For this review, take the finished solid that the model builds, in its own axes (mm). Face numbers are marked on the shaded views. A direction names the side the tool comes from. Give positions to 0.01 mm unless a question says otherwise; leave off trailing zeros. Order: outer loops, then holes, each group sorted by start corner. A loop starts at its lowest first (then second) coordinate and runs counter-clockwise, first axis right, second up. Notation, with made-up numbers: (-6, 8.25) -> (21, 8.25) arc R10 cw to (21, 18.25) -> close; hole circle Ø9 at (29, 70.5). An arc over 180 degrees is marked (long way). Return JSON: item names as keys, results as strings. Group by question number.
1) Insertion check: P1, Ø3.5, axis at x = -1.5, z = -1.5, coming from the +Y side; P2, Ø1.5, axis at y = 10.5, z = -13.5, coming from the -X side; P3, Ø2, axis at y = 7.5, z = -9.5, coming from the -X side; P4, Ø5, axis at y = 8.5, z = 4.5, coming from the -X side. Each pin has a flat end and moves straight along its axis. Give the tip position at first contact, or say it passes through.
2) The part is to be moulded in two halves that separate along Y. For the marked faces 6, 7 and 8, say which applies: released by +Y, released by -Y, zero draft, split by the parting line, or undercut.
3) Add section D-D (z = -7.5). Give the boundary of the cut face in (x, y), then the cut area to 3 significant figures.
4) For the marked faces 1, 2, 3, 4 and 5, list the 3-axis set-ups (+Z, -Z, +X, -X, +Y, -Y) from which the entire face can be reached by the end or side of a thin tool; tool diameter is ignored.
5) Add section C-C (x = 0). Give the boundary of the cut face in (y, z), then the cut area to 3 significant figures.
6) To check wall thickness, follow line 1 along X through (y, z) = (14.2, 0); line 2 along X through (y, z) = (4, 1.75); line 3 along Z through (x, y) = (0, 14.7). State the ranges of each line that lie inside material, in increasing order.
7) Add section A-A (z = 0). Give the boundary of the cut face in (x, y), then the cut area to 3 significant figures.
8) Add section B-B (y = 7.5). Give the boundary of the cut face in (x, z), then the cut area to 3 significant figures.
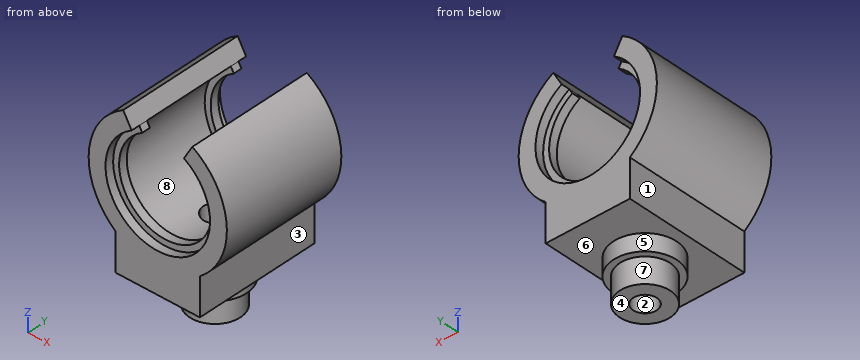
from build123d import *

# Parameters (mm, degrees)
SKETCH1_R               = 6.211279156
BOSS_EXTRUDE1_DEPTH     = 15
CUT_EXTRUDE1_DEPTH      = 21.332857777
CUT_EXTRUDE1_DEPTH_BACK = 21.332857777
BOSS_EXTRUDE3_DEPTH     = 1
SKETCH6_R               = 1.4
CUT_EXTRUDE2_DEPTH      = 10
SKETCH7_R               = 3.75
BOSS_EXTRUDE4_DEPTH     = 2
SKETCH8_R               = 3
BOSS_EXTRUDE5_DEPTH     = 3
CUT_EXTRUDE3_DEPTH      = 29.749810043
CUT_EXTRUDE3_DEPTH_BACK = 29.749810043
SKETCH9_R               = 1.4


with BuildPart() as part:
    # Sketch1 → Boss-Extrude1 (new body)
    with BuildSketch(Plane(origin=(0, 0, 0), x_dir=(1, 0, 0), z_dir=(0, 1, 0))):
        with BuildLine():
            Line((-5, 6.513455717), (-5, 11))
            Line((-5, 11), (5, 11))
            Line((5, 11), (5, 6.513455717))
            ThreePointArc((5, 6.513455717), (0, -8.211279156), (-5, 6.513455717))
        make_face()
        with Locations(Location((0, 0, 0), (0, 0, 270))):
            Circle(SKETCH1_R, mode=Mode.SUBTRACT)
    extrude(amount=BOSS_EXTRUDE1_DEPTH)

    # Sketch4 → Cut-Extrude1 (cut, two sides: drawn at the far end of the back side and taken through both)
    with BuildSketch(Plane(origin=(0, 15, 0), x_dir=(1, 0, 0), z_dir=(0, 1, 0)).offset(-CUT_EXTRUDE1_DEPTH_BACK)):
        with BuildLine():
            Line((-3.105639578, -5.379125539), (-4.105639578, -7.111176346))
            ThreePointArc((-4.105639578, -7.111176346), (0, -8.211279156), (4.105639578, -7.111176346))
            Line((4.105639578, -7.111176346), (3.105639578, -5.379125539))
            ThreePointArc((3.105639578, -5.379125539), (0, -6.211279156), (-3.105639578, -5.379125539))
        make_face()
    extrude(amount=CUT_EXTRUDE1_DEPTH + CUT_EXTRUDE1_DEPTH_BACK, mode=Mode.SUBTRACT)

    # Sketch5 → Boss-Extrude3 (add)
    with BuildSketch(Plane(origin=(0, 1, 0), x_dir=(-1, 0, 0), z_dir=(0, -1, 0))):
        with BuildLine():
            Line((3.105639578, -5.379125539), (2.749999992, -4.763139708))
            ThreePointArc((2.749999992, -4.763139708), (0, 5.499999985), (-2.749999992, -4.763139708))
            Line((-2.749999992, -4.763139708), (-3.105639578, -5.379125539))
            ThreePointArc((-3.105639578, -5.379125539), (0, 6.211279156), (3.105639578, -5.379125539))
        make_face()
    boss_extrude3 = extrude(amount=-BOSS_EXTRUDE3_DEPTH)

    # Mirror1: Boss-Extrude3 across plane
    add(boss_extrude3.mirror(Plane.ZX.offset(7.5)))

    # Sketch6 → Cut-Extrude2 (cut)
    with BuildSketch(Plane(origin=(0, 0, -11), x_dir=(-1, 0, 0), z_dir=(0, 0, -1))):
        with Locations((0, 7.5)):
            Circle(SKETCH6_R)
    extrude(amount=-CUT_EXTRUDE2_DEPTH, mode=Mode.SUBTRACT)

    # Sketch7 → Boss-Extrude4 (add)
    with BuildSketch(Plane(origin=(0, 0, -11), x_dir=(-1, 0, 0), z_dir=(0, 0, -1))):
        with Locations((0, 7.5)):
            Circle(SKETCH7_R)
    extrude(amount=BOSS_EXTRUDE4_DEPTH)

    # Sketch8 → Boss-Extrude5 (add)
    with BuildSketch(Plane(origin=(0, 0, -13), x_dir=(-1, 0, 0), z_dir=(0, 0, -1))):
        with Locations((0, 7.5)):
            Circle(SKETCH8_R)
    extrude(amount=BOSS_EXTRUDE5_DEPTH)

    # Sketch9 → Cut-Extrude3 (cut, two sides: drawn at the far end of the back side and taken through both)
    with BuildSketch(Plane(origin=(0, 0, -16), x_dir=(-1, 0, 0), z_dir=(0, 0, -1)).offset(-CUT_EXTRUDE3_DEPTH_BACK)):
        with Locations((0, 7.5)):
            Circle(SKETCH9_R)
    extrude(amount=CUT_EXTRUDE3_DEPTH + CUT_EXTRUDE3_DEPTH_BACK, mode=Mode.SUBTRACT)


solid = part.part
Evaluation:
{
 "1": {"P1": "through", "P2": "x = -2.85", "P3": "x = -5", "P4": "x = -7.96"},
 "2": {"face 6": "zero draft", "face 7": "split by the parting line", "face 8": "undercut"},
 "3": {"outline": "(-5, 0) -> (5, 0) -> (5, 15) -> (-5, 15) -> close; hole circle Ø2.8 at (0, 7.5)", "area": "144 mm^2"},
 "4": {"face 1": "-Z, -X, +Y, -Y", "face 2": "+Z, -Z", "face 3": "-Z, +X, +Y, -Y", "face 4": "-Z, +X, -X, +Y, -Y", "face 5": "-Z"},
 "5": {"outline": "(0, -11) -> (3.75, -11) -> (3.75, -13) -> (4.5, -13) -> (4.5, -16) -> (6.1, -16) -> (6.1, -6.21) -> (2, -6.21) -> (2, -5.5) -> (1, -5.5) -> (1, -6.21) -> (0, -6.21) -> close; (8.9, -16) -> (10.5, -16) -> (10.5, -13) -> (11.25, -13) -> (11.25, -11) -> (15, -11) -> (15, -6.21) -> (14, -6.21) -> (14, -5.5) -> (13, -5.5) -> (13, -6.21) -> (8.9, -6.21) -> close", "area": "78.8 mm^2"},
 "6": {"line 1": "-8.21 to -6.21, 6.21 to 8.21", "line 2": "-8.02 to -5.96, 5.96 to 8.02", "line 3": "-11 to -6.21"},
 "7": {"outline": "(-8.21, 0) -> (-6.21, 0) -> (-6.21, 1) -> (-5.5, 1) -> (-5.5, 2) -> (-6.21, 2) -> (-6.21, 13) -> (-5.5, 13) -> (-5.5, 14) -> (-6.21, 14) -> (-6.21, 15) -> (-8.21, 15) -> close; (5.5, 1) -> (6.21, 1) -> (6.21, 0) -> (8.21, 0) -> (8.21, 15) -> (6.21, 15) -> (6.21, 14) -> (5.5, 14) -> (5.5, 13) -> (6.21, 13) -> (6.21, 2) -> (5.5, 2) -> close", "area": "62.8 mm^2"},
 "8": {"outline": "(-5, -11) -> (-3.75, -11) -> (-3.75, -13) -> (-3, -13) -> (-3, -16) -> (-1.4, -16) -> (-1.4, -6.05) arc R6.21 cw to (-3.11, 5.38) -> (-4.11, 7.11) arc R8.21 ccw to (-5, -6.51) -> close; (1.4, -16) -> (3, -16) -> (3, -13) -> (3.75, -13) -> (3.75, -11) -> (5, -11) -> (5, -6.51) arc R8.21 ccw to (4.11, 7.11) -> (3.11, 5.38) arc R6.21 cw to (1.4, -6.05) -> close", "area": "114 mm^2"}
}
